Verification items for the finished model (mm, model axes). Give positions to 0.01 mm unless a question says otherwise; leave off trailing zeros. Write each loop counter-clockwise with the first axis right and the second up, starting at its lowest first coordinate (ties: lowest second). Pieces come first, ordered by that corner, then holes. Notation, with made-up numbers: (28.5, 38) -> (39.5, 38) arc R35 ccw to (39.5, 73) -> close; hole circle Ø3 at (-30, 37.25). An arc over 180 degrees is marked (long way). Use one line per item in the form item = value. Start each with the question number.
(1) Section check A-A, the plane x = -154.5. Record the cut outline in (y, z) (3 decimals).
(2) Scan lines: L1, parallel to Z at x = -154, y = 2; L2, parallel to Z at x = -168, y = -0.75; L3, parallel to Z at x = -156, y = 3.5. Record each from-to range of solid material in increasing order.
(3) Section check B-B, the plane y = -0.25. Record the cut outline in (x, z), plus the area to 3 significant figures.
(4) Section check C-C, the plane z = -101. Record the cut outline in (x, y).
(5) Depth check by flat-ended pin: pin 1 Ø1.5 at (y, z) = (3.5, -35) entering from -X; pin 2 Ø1 at (y, z) = (4, -121) entering from +X; pin 3 Ø3 at (y, z) = (-1, -110.5) entering from -X; pin 4 Ø4 at (x, z) = (-194.26, -17) entering from -Y. Enter the tip coordinate at first touch or a pass-through.
(6) Section check D-D, the plane x = -172.5. Record the cut outline in (y, z), plus the area to 3 significant figures.
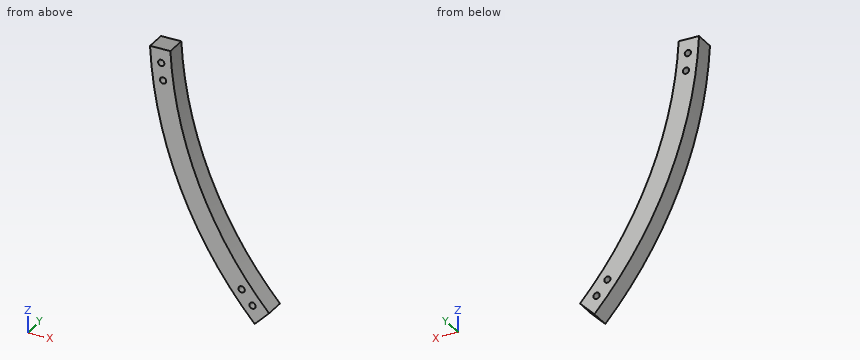
from build123d import *

# Parameters (mm, degrees)
BASE_DEPTH                 = 5
F_3_1_3_1_DIAMETER_HOLE1_D = 3.1


with BuildPart() as part:
    # Sketch1 → base (new, symmetric)
    with BuildSketch(Plane(origin=(0, 0, 0), x_dir=(1, 0, 0), z_dir=(0, 1, 0))):
        with BuildLine():
            Line((-141.235146462, 127.093010838), (-148.31553673, 134.173401106))
            ThreePointArc((-148.31553673, 134.173401106), (-184.775906502, 76.536686473), (-199.749843554, 10))
            Line((-199.749843554, 10), (-189.73665961, 10))
            ThreePointArc((-189.73665961, 10), (-175.537111177, 72.709852149), (-141.235146462, 127.093010838))
        make_face()
    extrude(amount=BASE_DEPTH, both=True)

    # Ø3.1 (3.1) Diameter Hole1 (through all)
    with Locations(Plane(origin=(0, 5, 0), x_dir=(1, 0, 0), z_dir=(0, 1, 0))):
        with Locations((-194.257966128, 16.995369836), (-149.378666408, 125.343583889), (-154.703901357, 118.708478657), (-193.331747968, 25.452607483)):
            Hole(F_3_1_3_1_DIAMETER_HOLE1_D / 2)


solid = part.part
Completed:
q1.outline = (-5, -127.003) -> (5, -127.003) -> (5, -120.245) -> (-5, -120.245) -> close; (-5, -117.172) -> (5, -117.172) -> (5, -110.588) -> (-5, -110.588) -> close
q2.L1 = -127.61 to -120.09, -117.33 to -111.28
q2.L2 = -108.52 to -88.75
q2.L3 = -125.16 to -119.56, -117.86 to -108.46
q3.outline = (-199.75, -10) arc R200 ccw to (-148.32, -134.17) -> (-141.24, -127.09) arc R190 cw to (-189.74, -10) -> close; hole circle Ø3.1 at (-194.26, -17); hole circle Ø3.1 at (-193.33, -25.45); hole circle Ø3.1 at (-154.7, -118.71); hole circle Ø3.1 at (-149.38, -125.34)
q3.area = 1,300 mm²
q4.outline = (-172.62, -5) -> (-160.93, -5) -> (-160.93, 5) -> (-172.62, 5) -> close
q5.pin_1 = -197.05
q5.pin_2 = -146.07
q5.pin_3 = -167.69
q5.pin_4 = -5
q6.outline = (-5, -101.21) -> (5, -101.21) -> (5, -79.65) -> (-5, -79.65) -> close
q6.area = 216 mm²
